Model file for the job. Use its own axes, mm. Give positions to 0.01 mm unless a question says otherwise; leave off trailing zeros. Loops run counter-clockwise (first coordinate to the right, second up) from the corner with the lowest first, then second, coordinate; pieces in that order, holes last. Notation, with made-up numbers: M 33.25,52 L 62.25,52 A30 cw 62.25,83 Z; hole C 89,-11.5 d7. An arc over 180 degrees is marked long. Use CSV: the item, a comma, the result in double quotes. Start each with the question number.
(1) Flat gauge pins, fed straight in: P1, Ø5, axis at x = 70, y = -51.5, coming from the -Z side; P2, Ø6, axis at x = 0, y = -15.875, coming from the -Z side. Where does each tip first touch, or does it go through?
(2) Two-plate mould, pull along Y, no slides. Class faces 1 (the face through (-2, 1, 3.175)), 2 (the face through (146.65, 64.76, 1.41)): pulls with the +Y half, pulls with the -Y half, needs draft (parallel to the pull), parting line crosses it, or undercut.
(3) Slice it at B-B on z = 2.5. State how many separate pieces and enclosed holes the cut face has, and give its area (3 significant figures).
(4) Wall check: line 1 along Y through (x, z) = (-146.05, 0.5) (3 decimals); line 2 along X through (y, z) = (-40, 1.55); line 3 along X through (y, z) = (-34.5, 0.25). Give the ranges that are in metal, low to high. Write a range as from..to.
(5) Slice it at A-A on x = 76. List the corners of the cut face in (y, z) (3 decimals), and give its area (3 significant figures).
Autodesk Inventor part; units mm, degrees
ref_plane "YZ Plane" through (0, 0, 0) normal (1, 0, 0) x (0, 1, 0)
ref_plane "XZ Plane" through (0, 0, 0) normal (0, 1, 0) x (-1, 0, 0)
ref_plane "XY Plane" through (0, 0, 0) normal (0, 0, 1) x (1, 0, 0)
sketch "Sketch1" plane through (0, 0, 0) normal (0, 0, 1) x (1, 0, 0)
  line L0 (-165.1, 69.85) -> (165.1, 69.85)
  line L1 (165.1, 69.85) -> (165.1, -69.85)
  line L2 (165.1, -69.85) -> (-165.1, -69.85)
  line L3 (-165.1, -69.85) -> (-165.1, 69.85)
  point P0 (0, 0)
  dimension "d0" = 139.7
  dimension "d1" = 330.2
  dimension "d2" = 69.85
  dimension "d3" = 165.1
extrude "Extrusion1" add sketch "Sketch1" along normal blind 3.175
sketch "Sketch2" plane through (0, 0, 3.175) normal (0, 0, 1) x (1, 0, 0)
  line L0 (0, -97.79) -> (0, 97.79) construction
  line L1 (-162.2078, 6.35) -> (163.5203, 6.35) construction
  line L2 (-165.1, 69.85) -> (165.1, 69.85)
  point P0 (0, 0)
  point P1 (-121.92, 6.35)
  point P2 (121.92, 6.35)
  dimension "d6" = 121.92
  dimension "d23" = 63.5
hole "Hole1" at (-121.92, 6.35, 3.175) at (121.92, 6.35, 3.175) direction (0, 0, -1) diameter 14.2875 end through all
sketch "Sketch4" plane through (0, 0, 3.175) normal (0, 0, 1) x (1, 0, 0)
  line L0 (-165.1, 69.85) -> (165.1, 69.85)
  line L1 (-165.1, -69.85) -> (-165.1, 69.85)
  line L2 (165.1, -69.85) -> (-165.1, -69.85)
  line L3 (165.1, 69.85) -> (165.1, -69.85)
  line L4 (-165.1, -15.875) -> (165.1, -15.875) construction
  line L5 (0, 69.85) -> (0, -69.85) construction
  line L6 (-146.05, 69.85) -> (-146.05, -69.85) construction
  line L7 (-165.1, 66.675) -> (165.1, 66.675) construction
  point P0 (0, 0)
  point P1 (-146.05, -15.875)
  point P2 (146.05, -15.875)
  point P3 (0, -15.875)
  point P4 (-146.05, -31.75)
  point P5 (-146.05, -57.15)
  point P6 (146.05, -31.75)
  point P7 (146.05, -57.15)
  point P8 (0, 66.675)
  point P9 (-146.05, 66.675)
  point P10 (146.05, 66.675)
  dimension "d24" = 85.725
  dimension "d49" = 12.7
  dimension "d50" = 25.4
  dimension "d51" = 3.175
  dimension "d58" = 146.05
hole "Hole3" at (-146.05, -15.875, 3.175) at (146.05, -15.875, 3.175) at (0, -15.875, 3.175) at (-146.05, -31.75, 3.175) at (-146.05, -57.15, 3.175) at (146.05, -31.75, 3.175) at (146.05, -57.15, 3.175) at (-146.05, 66.675, 3.175) at (146.05, 66.675, 3.175) at (0, 66.675, 3.175) direction (0, 0, -1) diameter 3.81 end through all countersink diameter 7.0866 countersink angle 82
sketch "Sketch5" plane through (0, 0, 3.175) normal (0, 0, 1) x (1, 0, 0)
  line L0 (-83.1, -33.2) -> (-38.1, -33.2)
  line L1 (-38.1, -33.2) -> (-38.1, -55.7)
  line L2 (-38.1, -55.7) -> (-83.1, -55.7)
  line L3 (-83.1, -55.7) -> (-83.1, -33.2)
  line L4 (0, -97.79) -> (0, 97.79) construction
  line L5 (165.1, -69.85) -> (-165.1, -69.85) construction
  line L6 (-155.899, -44.45) -> (168.0806, -44.45) construction
  line L7 (-121.2, -34.925) -> (-108.5, -34.925)
  line L8 (-108.5, -34.925) -> (-108.5, -53.975)
  line L9 (-108.5, -53.975) -> (-121.2, -53.975)
  line L10 (-121.2, -53.975) -> (-121.2, -34.925)
  line L11 (83.1, -33.2) -> (38.1, -33.2)
  line L12 (38.1, -33.2) -> (38.1, -55.7)
  line L13 (38.1, -55.7) -> (83.1, -55.7)
  line L14 (83.1, -55.7) -> (83.1, -33.2)
  line L15 (121.2, -34.925) -> (108.5, -34.925)
  line L16 (108.5, -34.925) -> (108.5, -53.975)
  line L17 (108.5, -53.975) -> (121.2, -53.975)
  line L18 (121.2, -53.975) -> (121.2, -34.925)
  point P0 (0, 0)
  dimension "d33" = 45
  dimension "d36" = 38.1
  dimension "d53" = 25.4
  dimension "d54" = 22.5
  dimension "d55" = 12.7
  dimension "d56" = 19.05
  dimension "d57" = 25.4
extrude "Extrusion2" cut sketch "Sketch5" against normal up to next
fillet "Fillet1" radius 1.5875 16 edges at (-121.2, -53.975, 1.5875) (-83.1, -55.7, 1.5875) (38.1, -55.7, 1.5875) (108.5, -53.975, 1.5875) (-108.5, -53.975, 1.5875) (-38.1, -55.7, 1.5875) (83.1, -55.7, 1.5875) (121.2, -53.975, 1.5875) (121.2, -34.925, 1.5875) (83.1, -33.2, 1.5875) (-38.1, -33.2, 1.5875) (-108.5, -34.925, 1.5875) (108.5, -34.925, 1.5875) (38.1, -33.2, 1.5875) (-83.1, -33.2, 1.5875) (-121.2, -34.925, 1.5875)
properties part number "J001397" material "ALUMINUM, 6061-T651"
Reply:
1,P1,"passes through"
1,P2,"stops at z = 0"
2,face 1,"needs draft"
2,face 2,"undercut"
3,separate pieces,"1"
3,enclosed holes,"16"
3,area,"43,000 mm^2"
4,line 1,"y = -69.85..-59.055, -55.245..-33.655, -29.845..-17.78, -13.97..64.77, 68.58..69.85"
4,line 2,"x = -165.1..-121.2, -108.5..-83.1, -38.1..38.1, 83.1..108.5, 121.2..165.1"
4,line 3,"x = -165.1..-83.07, -38.13..38.13, 83.07..165.1"
5,outline,"M -69.85,0 L -55.7,0 L -55.7,3.175 L -69.85,3.175 Z; M -33.2,0 L 69.85,0 L 69.85,3.175 L -33.2,3.175 Z"
5,area,"372 mm^2"
